Geometry check sheet. Reference: the model listing, model coordinates, mm. Give positions to 0.01 mm unless a question says otherwise; leave off trailing zeros. Write each loop counter-clockwise with the first axis right and the second up, starting at its lowest first coordinate (ties: lowest second). Pieces come first, ordered by that corner, then holes.
(1) Cross-section at D-D (y = 100.5). Record the boundary of the cut face in (x, z) (3 decimals), and give its area (3 significant figures).
(2) Depth check by flat-ended pin: P1, Ø2.5, axis at x = -70, y = 58.71, coming from the +Z side; P2, Ø1, axis at y = 92, z = 2.5, coming from the -X side; P3, Ø1.5, axis at x = 41, z = 0.5, coming from the +Y side. Enter the tip coordinate at first touch or a pass-through.
(3) Cross-section at B-B (x = 0). Record the boundary of the cut face in (y, z) (3 decimals).
(4) Thickness scan on line 1 along X through (y, z) = (117.5, 0.75); line 2 along Y through (x, z) = (-10, 1); line 3 along Y through (x, z) = (25, 1.25). Record the ranges inside material, lowest first.
(5) Mould release check, pull along X, two halves, no side actions. Record for faces 1 (the cylindrical face through (62, 19.52, 1.57)), 2 (the cylindrical face through (67.482, -117.871, 1.61)), 3 (the flat face through (-57.995, 89.501, 1.565)): +X half, -X half, draft (parallel to the pull), parting line (faces both ways), or undercut.
(6) Cross-section at A-A (y = -56). Record the boundary of the cut face in (x, z) (3 decimals).
(7) Cross-section at C-C (z = 2.55). Record the boundary of the cut face in (x, y) (1 decimal), and give its area (3 significant figures).
```python
from build123d import *

# Parameters (mm, degrees)
F0_R     = 65
F1_DEPTH = 3.175
F2_R     = 25
F3_R     = 1.5875
F4_DEPTH = 3.176


with BuildPart() as f1:
    # F0 (on Top) → F1 (new body)
    with BuildSketch(Plane.XY):
        Polygon((-75, 60.048095), (-75, -125), (75, -125), (75, 60.048095), (37.5, 125), (-37.5, 125), align=None)
        Circle(F0_R, mode=Mode.SUBTRACT)
    extrude(amount=F1_DEPTH)

    # F2
    f2_edges = [f1.edges().sort_by_distance(p)[0] for p in [
        (-75, -125, 1.5875),
        (75, -125, 1.5875),
        (-37.5, 125, 1.5875),
        (-75, 60.048095, 1.5875),
        (75, 60.048095, 1.5875),
        (37.5, 125, 1.5875),
    ]]
    fillet(f2_edges, radius=F2_R)

    # F3 (on face) → F4 (cut, through all)
    with BuildSketch(Plane.XY.offset(3.175)):
        with Locations((-33.169873, 117.5)):
            Circle(F3_R)
        with Locations((33.169873, 117.5)):
            Circle(F3_R)
        with Locations((70, 58.708349)):
            Circle(F3_R)
        with Locations((-70, 58.708349)):
            Circle(F3_R)
        with Locations((-64.142136, -114.142136)):
            Circle(F3_R)
        with Locations((64.142136, -114.142136)):
            Circle(F3_R)
    extrude(amount=-F4_DEPTH, mode=Mode.SUBTRACT)


solid = f1.part
```
Reply:
1. outline: (-51.645, 0) - (51.645, 0) - (51.645, 3.175) - (-51.645, 3.175) - close
1. area: 328 mm2
2. P1: passes through
2. P2: stops at x = -56.84
2. P3: stops at y = 118.16
3. outline: (-125, 0) - (-65, 0) - (-65, 3.175) - (-125, 3.175) - close; (65, 0) - (125, 0) - (125, 3.175) - (65, 3.175) - close
4. line 1: x = -40.92 to -34.76, -31.58 to 31.58, 34.76 to 40.92
4. line 2: y = -125 to -64.23, 64.23 to 125
4. line 3: y = -125 to -60, 60 to 124.93
5. face 1: undercut
5. face 2: +X half
5. face 3: -X half
6. outline: (-75, 0) - (-33, 0) - (-33, 3.175) - (-75, 3.175) - close; (33, 0) - (75, 0) - (75, 3.175) - (33, 3.175) - close
7. outline: (-75, -100) arc R25 ccw to (-50, -125) - (50, -125) arc R25 ccw to (75, -100) - (75, 53.3) arc R25 ccw to (71.7, 65.8) - (44.7, 112.5) arc R25 ccw to (23.1, 125) - (-23.1, 125) arc R25 ccw to (-44.7, 112.5) - (-71.7, 65.8) arc R25 ccw to (-75, 53.3) - close; hole circle Ø3.2 at (-70, 58.7); hole circle Ø3.2 at (-64.1, -114.1); hole circle Ø130 at (0, 0); hole circle Ø3.2 at (-33.2, 117.5); hole circle Ø3.2 at (33.2, 117.5); hole circle Ø3.2 at (64.1, -114.1); hole circle Ø3.2 at (70, 58.7)
7. area: 21,400 mm2
